from build123d import *

# Parameters (mm, degrees)
SKETCH1_R           = 12.7
SKETCH1_W           = 98
SKETCH1_H           = 16
BOSS_EXTRUDE1_DEPTH = 22
BOSS_EXTRUDE1_DRAFT = -8
SKETCH2_R           = 12.7
SKETCH2_W           = 56
SKETCH2_H           = 25.6
SKETCH2_W_2         = 46
SKETCH2_H_2         = 46
SKETCH2_W_3         = 74
SKETCH2_H_3         = 58
SKETCH2_W_4         = 24
BOSS_EXTRUDE2_DEPTH = 48
BOSS_EXTRUDE2_DRAFT = -4
SKETCH3_R           = 16
SKETCH3_R_2         = 12.7
SKETCH3_W           = 6
SKETCH3_H           = 29
BOSS_EXTRUDE3_DEPTH = 66


with BuildPart() as part:
    # Sketch1 → Boss-Extrude1 (with draft: the straight prism first)
    with BuildSketch(Plane.XY):
        Polygon((-78, 109), (-109, 78), (-109, -78), (-78, -109), (78, -109), (109, -78), (109, 78), (78, 109), align=None)
        with Locations((-45, -14.5)):
            Circle(SKETCH1_R, mode=Mode.SUBTRACT)
        with Locations((45, -14.5)):
            Circle(SKETCH1_R, mode=Mode.SUBTRACT)
        with Locations((0, 94)):
            Rectangle(SKETCH1_W, SKETCH1_H, mode=Mode.SUBTRACT)
    extrude(amount=BOSS_EXTRUDE1_DEPTH)
    # Boss-Extrude1: the draft: its side faces are tilted about the plane it starts from
    boss_extrude1_sides = [part.faces().sort_by_distance(p)[0] for p in [
        (-93.5, 93.5, 11),
        (-109, 0, 11),
        (-93.5, -93.5, 11),
        (0, -109, 11),
        (93.5, -93.5, 11),
        (109, 0, 11),
        (93.5, 93.5, 11),
        (0, 109, 11),
        (-57.7, -14.5, 11),
        (32.3, -14.5, 11),
        (-49, 94, 11),
        (0, 102, 11),
        (49, 94, 11),
        (0, 86, 11),
    ]]
    draft(boss_extrude1_sides, Plane.XY, BOSS_EXTRUDE1_DRAFT)


with BuildPart() as boss_extrude2_tool:
    # Sketch2 → Boss-Extrude2 (with draft: the straight prism first)
    with BuildSketch(Plane.XY):
        Polygon((-74, 104), (-104, 74), (-104, -74), (-74, -104), (74, -104), (104, -74), (104, 74), (74, 104), align=None)
        with Locations((-45, -14.5)):
            Circle(SKETCH2_R, mode=Mode.SUBTRACT)
        with Locations((45, -14.5)):
            Circle(SKETCH2_R, mode=Mode.SUBTRACT)
        with Locations((-45, 16.5)):
            Rectangle(SKETCH2_W, SKETCH2_H, mode=Mode.SUBTRACT)
        with Locations((45, 16.5)):
            Rectangle(SKETCH2_W, SKETCH2_H, mode=Mode.SUBTRACT)
        with Locations((0, 57)):
            Rectangle(SKETCH2_W_2, SKETCH2_H_2, mode=Mode.SUBTRACT)
        with Locations((0, -63)):
            Rectangle(SKETCH2_W_3, SKETCH2_H_3, mode=Mode.SUBTRACT)
        with Locations((-58, -58)):
            Rectangle(SKETCH2_W_4, SKETCH2_H_2, mode=Mode.SUBTRACT)
        with Locations((58, -58)):
            Rectangle(SKETCH2_W_4, SKETCH2_H_2, mode=Mode.SUBTRACT)
    extrude(amount=BOSS_EXTRUDE2_DEPTH)
    # Boss-Extrude2: the draft: its side faces are tilted about the plane it starts from
    boss_extrude2_sides = [boss_extrude2_tool.faces().sort_by_distance(p)[0] for p in [
        (-89, 89, 24),
        (-104, 0, 24),
        (-89, -89, 24),
        (0, -104, 24),
        (89, -89, 24),
        (104, 0, 24),
        (89, 89, 24),
        (0, 104, 24),
        (-57.7, -14.5, 24),
        (32.3, -14.5, 24),
        (-73, 16.5, 24),
        (-45, 29.3, 24),
        (-17, 16.5, 24),
        (-45, 3.7, 24),
        (17, 16.5, 24),
        (45, 29.3, 24),
        (73, 16.5, 24),
        (45, 3.7, 24),
        (-23, 57, 24),
        (0, 80, 24),
        (23, 57, 24),
        (0, 34, 24),
        (-37, -63, 24),
        (0, -34, 24),
        (37, -63, 24),
        (0, -92, 24),
        (-70, -58, 24),
        (-58, -35, 24),
        (-46, -58, 24),
        (-58, -81, 24),
        (46, -58, 24),
        (58, -35, 24),
        (70, -58, 24),
        (58, -81, 24),
    ]]
    draft(boss_extrude2_sides, Plane.XY, BOSS_EXTRUDE2_DRAFT)


with BuildPart() as part_1:
    add(part.part)

    # Boss-Extrude2: add boss_extrude2_tool
    add(boss_extrude2_tool.part)

    # Sketch3 → Boss-Extrude3 (add)
    # profile 1 of 4: a face of its own
    with BuildSketch(Plane.XY):
        with Locations(Location((-45, -14.5, 0), (0, 0, 180))):
            Circle(SKETCH3_R)
        with Locations(Location((-45, -14.5, 0), (0, 0, 180))):
            Circle(SKETCH3_R_2, mode=Mode.SUBTRACT)
    # profile 2 of 4: a face of its own
    with BuildSketch(Plane.XY):
        with Locations(Location((45, -14.5, 0), (0, 0, 180))):
            Circle(SKETCH3_R)
        with Locations(Location((45, -14.5, 0), (0, 0, 180))):
            Circle(SKETCH3_R_2, mode=Mode.SUBTRACT)
    # profile 3 of 4: a face of its own
    with BuildSketch(Plane.XY):
        with Locations((-76, 16.5)):
            Rectangle(SKETCH3_W, SKETCH3_H)
    # profile 4 of 4: a face of its own
    with BuildSketch(Plane.XY):
        with Locations((76, 16.5)):
            Rectangle(SKETCH3_W, SKETCH3_H)
    extrude(amount=BOSS_EXTRUDE3_DEPTH)


solid = part_1.part
Geometry check sheet. Reference: the model listing, model coordinates, mm. A direction names the side the tool comes from. Give positions to 0.01 mm unless a question says otherwise; leave off trailing zeros. Write each loop counter-clockwise with the first axis right and the second up, starting at its lowest first coordinate (ties: lowest second). Pieces come first, ordered by that corner, then holes. Notation, with made-up numbers: M 82.25,-39.5 L 95.25,-39.5 A23 cw 95.25,-15.5 Z; hole C -32.5,37 d8. An arc over 180 degrees is marked long. One line per question, with ' | ' between items.
1. Scan lines: line 1 along X through (y, z) = (-14, 57); line 2 along Y through (x, z) = (-51.5, 35); line 3 along X through (y, z) = (4, 62.5). Record each from-to range of solid material in increasing order. Write a range as from..to.
Ans:
line 1: -60.99..-57.69, -32.31..-29.01, 29.01..32.31, 57.69..60.99 | line 2: -106.45..-78.55, -37.45..-22.43, -6.57..6.15, 26.85..106.45 | line 3: -79..-73, 73..79
2. Cross-section at C-C (z = 8). Enter the section's corners in (x, y), plus the area to 3 significant figures.
Ans:
outline: M -110.12,-78.47 L -78.47,-110.12 L 78.47,-110.12 L 110.12,-78.47 L 110.12,78.47 L 78.47,110.12 L -78.47,110.12 L -110.12,78.47 Z; hole C -45,-14.5 d23.15; hole C 45,-14.5 d23.15 | area: 45,700 mm2
3. Cross-section at D-D (y = -71). Enter the section's corners in (x, z), plus the area to 3 significant figures.
Ans:
outline: M -112.09,22 L -109,0 L 109,0 L 112.09,22 L 105.54,22 L 107.36,48 L 66.64,48 L 68.46,22 L 47.54,22 L 49.36,48 L 33.64,48 L 35.46,22 L -35.46,22 L -33.64,48 L -49.36,48 L -47.54,22 L -68.46,22 L -66.64,48 L -107.36,48 L -105.54,22 Z | area: 7,610 mm2
4. Cross-section at A-A (y = 70). Enter the section's corners in (x, z), plus the area to 3 significant figures.
Ans:
outline: M -112.09,22 L -109,0 L 109,0 L 112.09,22 L 105.54,22 L 107.36,48 L 19.64,48 L 21.46,22 L -21.46,22 L -19.64,48 L -107.36,48 L -105.54,22 Z | area: 9,330 mm2
5. Gauge pin test, flat ends, axial feed: pin 1 (16.5 mm diameter, centred on x = -56, y = -66, fed in from +Z); pin 2 (2 mm diameter, centred on y = 0.5, z = 57, fed in from +X); pin 3 (11.5 mm diameter, centred on x = 40.5, y = 19.5, fed in from +Z). Record the tip position at first contact, or that the pin passes through.
Ans:
pin 1: z = 48 | pin 2: x = 52.75 | pin 3: z = 22
6. Cross-section at B-B (z = 31). Count the separate pieces of the cut face and the enclosed holes in it, plus the area to 3 significant figures.
Ans:
separate pieces: 1 | enclosed holes: 8 | area: 33,100 mm2
7. Set-up check for faces 4 (the face through (76, 2, 57)), 5 (the face through (90.498, -90.945, 34.818)), 6 (the face through (-0.496, -89.565, 34.818)): record each of +Z, -Z, +X, -X, +Y, -Y from which the full face is reachable in a straight line by a thin tool's end or side.
Ans:
face 4: +Z, +X, -X, -Y | face 5: +X, -Y | face 6: none
8. Mould release check, pull along Y, two halves, no side actions. Record for faces 1 (the face through (57.697, -4.764, 56.874)), 2 (the face through (94.348, -94.808, 10.846)), 3 (the face through (34.565, -63.384, 34.818)): released by +Y, released by -Y, zero draft, split by the parting line, or undercut.
Ans:
face 1: split by the parting line | face 2: released by -Y | face 3: undercut
